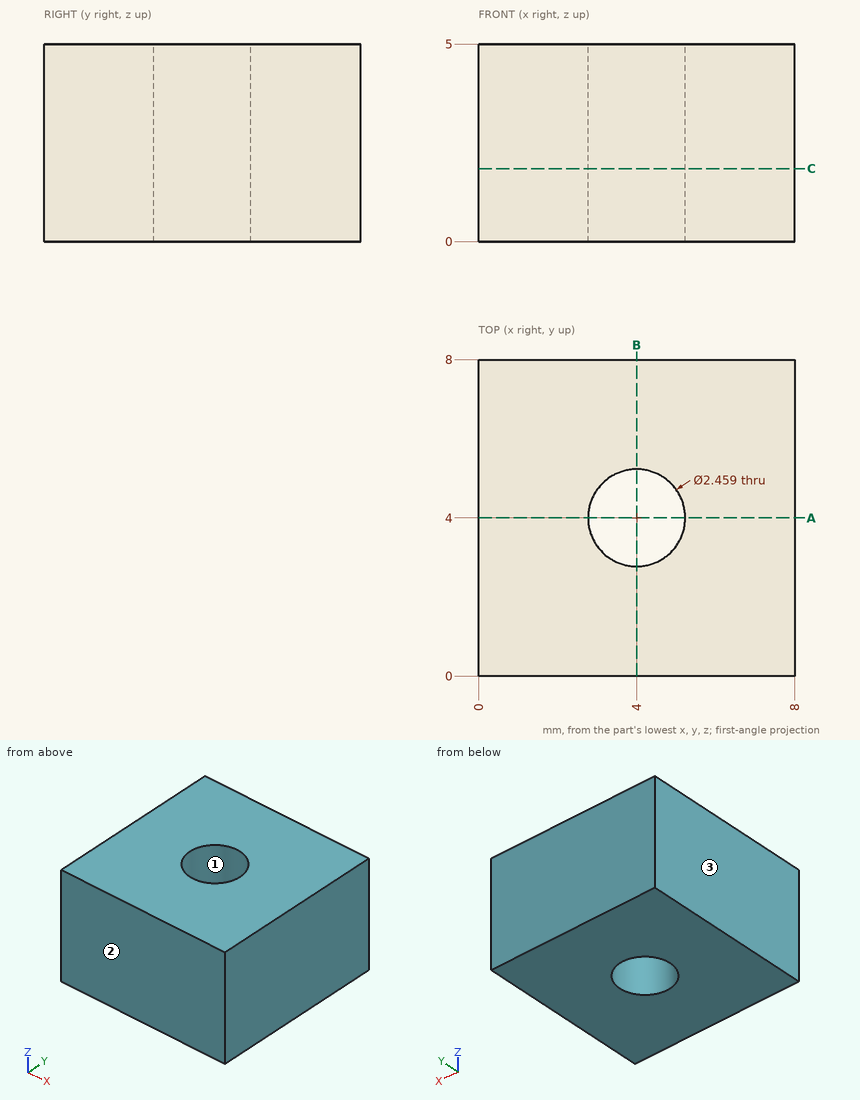
The figure shows three views and two pictorial views of one solid part (mm, origin at its lowest corner). Answer the questions. Give positions to 0.01 mm unless a question says otherwise; leave off trailing zeros. Write each loop counter-clockwise with the first axis right and the second up, starting at its lowest first coordinate (ties: lowest second). Pieces come first, ordered by that corner, then holes. Notation, with made-up numbers: (74, 0) -> (117, 0) arc R20 ccw to (117, 28) -> close; hole circle Ø9 at (60.25, 58.5). An arc over 180 degrees is marked (long way). Answer as a JSON object with one key per item and string values.
1) A flat-ended cylindrical pin translates along its axis: pin 1 Ø1.5 at (x, y) = (3.5, 1) entering from -Z. Find the tip coordinate at first contact, or state that the pin passes through.
Findings below:
{"pin 1": "stops at z = 0"}
2) Straight lines are drawn through the part: probe 1 along Y at (x, z) = (4, 3.2); probe 2 along X at (y, z) = (4.75, 2.9). For each, find the intervals that lie inside material, in ascending order. Write a range as from..to.
Findings below:
{"probe 1": "y = 0..2.77, 5.23..8", "probe 2": "x = 0..3.03, 4.97..8"}
3) For a pull along Y with two mould halves and no side action, classify the marked faces 1, 2 and 3 as pulls with the +Y half, pulls with the -Y half, needs draft (parallel to the pull), parting line crosses it, or undercut.
Findings below:
{"face 1": "undercut", "face 2": "pulls with the -Y half", "face 3": "needs draft"}
4) Section C-C on z = 1.85 is taken. Write down the section's boundary in (x, y), then the cut area to 3 significant figures.
Findings below:
{"outline": "(0, 0) -> (8, 0) -> (8, 8) -> (0, 8) -> close; hole circle Ø2.46 at (4, 4)", "area": "59.3 mm^2"}
5) Section A-A on y = 4 is taken. Write down the section's boundary in (x, z), then the cut area to 3 significant figures.
Findings below:
{"outline": "(0, 0) -> (2.77, 0) -> (2.77, 5) -> (0, 5) -> close; (5.23, 0) -> (8, 0) -> (8, 5) -> (5.23, 5) -> close", "area": "27.7 mm^2"}
